Work out the finished part from the listing and answer in its coordinate system (mm). A direction names the side the tool comes from. Give positions to 0.01 mm unless a question says otherwise; leave off trailing zeros. Loops run counter-clockwise (first coordinate to the right, second up) from the corner with the lowest first, then second, coordinate; pieces in that order, holes last. Notation, with made-up numbers: (59.5, 81.5) -> (101.5, 81.5) arc R7 cw to (101.5, 90.5) -> close; hole circle Ø3 at (61, 33.5). An arc over 180 degrees is marked (long way). Answer as CSV lines item,"result". Start each with the question number.
1. Determine the mould class of faces 1 (the face through (0, 30, -1)), 2 (the face through (51.815, 12.379, 2.218)), 3 (the face through (-73, 0, 10)) for opening direction Y: +Y half, -Y half, draft (parallel to the pull), parting line (faces both ways), or undercut.
2. Find the intervals of material crossed by line 1 along Y through (x, z) = (-50.5, 2.5); line 2 along X through (y, z) = (-19, -1.05); line 3 along X through (y, z) = (9, -0.9), in increasing order.
3. Flat-ended cylindrical pins translate along their axes: pin 1 Ø21.5 at (x, y) = (-58, -13) entering from +Z; pin 2 Ø0.6 at (x, y) = (-71.5, 26.5) entering from +Z; pin 3 Ø2 at (x, y) = (26, 8) entering from +Z. Find the tip coordinate at first contact, or state that the pin passes through.
4. A tool of negligible diameter and unlimited length cuts with its end or side. For faces 4 (the face through (53.42, -23.88, 2.22)), 5 (the face through (-59.247, 8.857, -0.521)), 6 (the face through (53, -18, 4.5)), from which of +Z, -Z, +X, -X, +Y, -Y can it reach the whole face along a straight path? Write none if from no direction.
5. Find section D-D, the plane x = -12.5. Give the vertices of the cut face in (y, z).
6. Find section A-A, the plane y = -19. Count the separate pieces of the cut face and the enclosed holes in it, and give its area (3 significant figures).
7. Find section B-B, the plane y = 16.5. Give the vertices of the cut face in (x, z).
8. Find section C-C, the plane z = 11.5. Give the vertices of the cut face in (x, y), and give its area (3 significant figures).
from build123d import *

# Parameters (mm, degrees)
F0_W            = 142
F0_H            = 60
F0_R            = 5
F1_DEPTH        = 19
F2_T            = 2
F3_T1_DEPTH     = 31
F4_W            = 6
F4_H            = 2
F4_W_2          = 2
F4_H_2          = 6
F5_DEPTH        = 3
F6_W            = 5
F6_H            = 6
F6_W_2          = 6
F6_H_2          = 5
F7_DEPTH        = 2
F7_TAPER        = 8
F8_R            = 1
F9_DEPTH        = 4.5
F11_D           = 3.3
F11_CBORE_D     = 6.5
F11_CBORE_DEPTH = 3


# Not quite as in the source:
# - a fillet or chamfer that OpenCascade refuses, or shapes differently, is made with other operations: its cross-section is extruded or revolved along the edge and cut away or added
# - a feature names something its author has since deleted; it is built from what else it names


with BuildPart() as f1:
    # F0 (on Top) → F1 (new body)
    with BuildSketch(Plane.XY):
        Rectangle(F0_W, F0_H)
        with Locations((-50.5, -19)):
            Circle(F0_R, mode=Mode.SUBTRACT)
        with Locations((54.5, -19)):
            Circle(F0_R, mode=Mode.SUBTRACT)
        with Locations((-56, 9)):
            Circle(F0_R, mode=Mode.SUBTRACT)
        with Locations((55.5, 9)):
            Circle(F0_R, mode=Mode.SUBTRACT)
        with Locations((-56, 9)):
            Circle(F0_R)
        with Locations((-50.5, -19)):
            Circle(F0_R)
        with Locations((54.5, -19)):
            Circle(F0_R)
        with Locations((55.5, 9)):
            Circle(F0_R)
    extrude(amount=F1_DEPTH)

    # F2
    f2_openings = [f1.faces().sort_by_distance(p)[0] for p in [
        (0, 0, 19),
        (0, 30, 9.5),
    ]]
    offset(amount=F2_T, openings=f2_openings, kind=Kind.INTERSECTION)

    # F3: fillet of radius 2 on 2 edges, made by hand

    # F3_s2 → F3_t1 (cut)
    with BuildSketch(Plane.XY.offset(-7)):
        with BuildLine():
            ThreePointArc((-71, -32), (-72.4142135624, -31.4142135624), (-73, -30))
            Line((-73, -30), (-73, -32))
            Line((-73, -32), (-71, -32))
        make_face()
        with BuildLine():
            ThreePointArc((71, -32), (72.4142135624, -31.4142135624), (73, -30))
            Line((73, -30), (73, -32))
            Line((73, -32), (71, -32))
        make_face()
    extrude(amount=F3_T1_DEPTH, mode=Mode.SUBTRACT)

    # F4 (on face) → F5 (join)
    with BuildSketch(Plane.XY.offset(19)):
        with Locations((-43, -31)):
            Rectangle(F4_W, F4_H)
        with Locations((-72, 21)):
            Rectangle(F4_W_2, F4_H_2)
        with Locations((72, 21)):
            Rectangle(F4_W_2, F4_H_2)
        with Locations((43, -31)):
            Rectangle(F4_W, F4_H)
    extrude(amount=F5_DEPTH)

    # F6 (on face) → F7 (join)
    with BuildSketch(Plane.XY.offset(22)):
        with Locations((-73.5, 21)):
            Rectangle(F6_W, F6_H)
        with Locations((-43, -32.5)):
            Rectangle(F6_W_2, F6_H_2)
        with Locations((43, -32.5)):
            Rectangle(F6_W_2, F6_H_2)
        with Locations((73.5, 21)):
            Rectangle(F6_W, F6_H)
    extrude(amount=F7_DEPTH, taper=F7_TAPER)

    # F8
    f8_edges = [f1.edges().sort_by_distance(p)[0] for p in [
        (-71.281082, 21, 24),
        (-43, -30.281082, 24),
        (43, -30.281082, 24),
        (71.281082, 21, 24),
    ]]
    fillet(f8_edges, radius=F8_R)

    # F0 (on Top) → F9 (join)
    with BuildSketch(Plane.XY):
        with Locations((-56, 9)):
            Circle(F0_R)
        with Locations((55.5, 9)):
            Circle(F0_R)
        with Locations((54.5, -19)):
            Circle(F0_R)
        with Locations((-50.5, -19)):
            Circle(F0_R)
    extrude(amount=F9_DEPTH)

    # F11 (through all)
    with Locations(Plane(origin=(0, 0, -2), x_dir=(1, 0, 0), z_dir=(0, 0, -1))):
        with Locations((-50.5, 19), (-56, -9), (55.5, -9), (54.5, 19)):
            CounterBoreHole(F11_D / 2, F11_CBORE_D / 2, F11_CBORE_DEPTH)


solid = f1.part
Resolved:
1,face 1,"+Y half"
1,face 2,"undercut"
1,face 3,"draft"
2,line 1,"y = -32 to -30, -24 to -20.65, -17.35 to -14"
2,line 2,"x = -73 to -53.75, -47.25 to 51.25, 57.75 to 73"
2,line 3,"x = -73 to -59.25, -52.75 to 52.25, 58.75 to 73"
3,pin 1,"stops at z = 4.5"
3,pin 2,"stops at z = 19"
3,pin 3,"stops at z = 0"
4,face 4,"+Z"
4,face 5,"-Z"
4,face 6,"+Z, +Y"
5,outline,"(-32, -2) -> (30, -2) -> (30, 0) -> (-30, 0) -> (-30, 19) -> (-32, 19) -> close"
6,separate pieces,"3"
6,enclosed holes,"0"
6,area,"396 mm^2"
7,outline,"(-73, -2) -> (73, -2) -> (73, 19) -> (71, 19) -> (71, 0) -> (-71, 0) -> (-71, 19) -> (-73, 19) -> close"
8,outline,"(-73, -30) arc R2 ccw to (-71, -32) -> (71, -32) arc R2 ccw to (73, -30) -> (73, 30) -> (71, 30) -> (71, -30) -> (-71, -30) -> (-71, 30) -> (-73, 30) -> close"
8,area,"530 mm^2"
